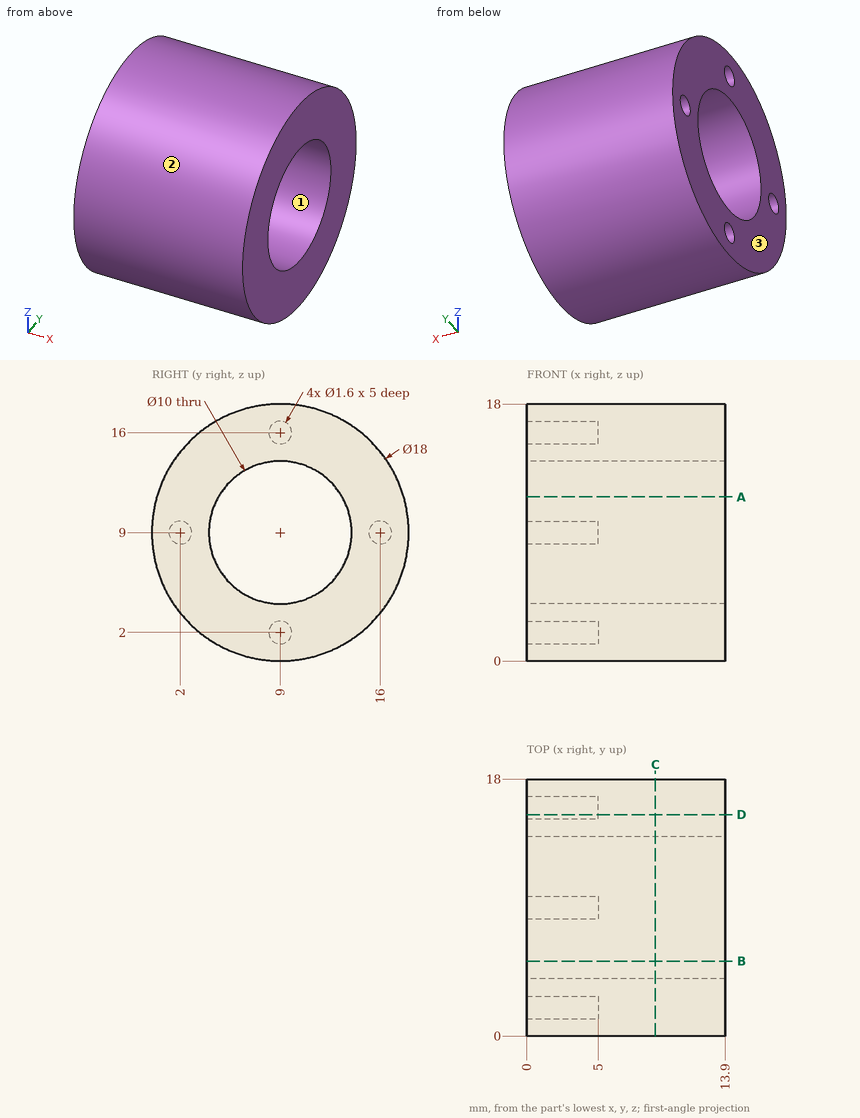
Part print with two shaded views. Sizes in mm from the minimum x, y, z corner. Round coordinates to 2 decimals unless told otherwise and drop trailing zeros. Order: outer loops, then holes, each group sorted by start corner. A loop starts at its lowest first (then second) coordinate and runs counter-clockwise, first axis right, second up. Notation, with made-up numbers: M 20,82.5 L 68,82.5 A26 ccw 68,96.5 Z; hole C -14.5,60 d8. An arc over 180 degrees is marked long. Put each result on its own line as item: value. Start each with the question number.
1. Slice it at A-A on z = 11.5. List the corners of the cut face in (x, y), then the cut area to 3 significant figures.
2. Slice it at C-C on x = 9. List the corners of the cut face in (y, z).
3. Two-plate mould, pull along Z, no slides. Class the marked faces 1, 2 and 3: +Z half, -Z half, draft (parallel to the pull), parting line (faces both ways), or undercut.
4. Slice it at B-B on y = 5.25. List the corners of the cut face in (x, z), then the cut area to 3 significant figures.
5. Drill centre lines: probe 1 along Z at (x, y) = (8.5, 5.25); probe 2 along Z at (x, y) = (12.5, 11). Where is each one in solid material? Low to high. Write a range as [from, to].
6. Slice it at D-D on y = 15.5. List the corners of the cut face in (x, z).
7. Drop flat-ended pins along their axis: pin 1 (0.5 mm diameter, centred on y = 15.5, z = 9, fed in from -X); pin 2 (2 mm diameter, centred on x = 6, y = 5, fed in from +Z); pin 3 (3 mm diameter, centred on x = 10.5, y = 2.5, fed in from +Z). Give the stop position or say it passes through.
Findings:
1. outline: M 0,0.35 L 13.9,0.35 L 13.9,4.67 L 0,4.67 Z; M 0,13.33 L 13.9,13.33 L 13.9,17.65 L 0,17.65 Z
1. area: 120 mm2
2. outline: C 9,9 d18; hole C 9,9 d10
3. face 1: undercut
3. face 2: parting line
3. face 3: draft
4. outline: M 0,0.82 L 13.9,0.82 L 13.9,5.69 L 0,5.69 Z; M 0,12.31 L 13.9,12.31 L 13.9,17.18 L 0,17.18 Z
4. area: 136 mm2
5. probe 1: [0.82, 5.69], [12.31, 17.18]
5. probe 2: [0.23, 4.42], [13.58, 17.77]
6. outline: M 0,2.78 L 13.9,2.78 L 13.9,15.22 L 0,15.22 L 0,9.62 L 5,9.62 L 5,8.38 L 0,8.38 Z
7. pin 1: x = 5
7. pin 2: z = 17.49
7. pin 3: z = 16.48
